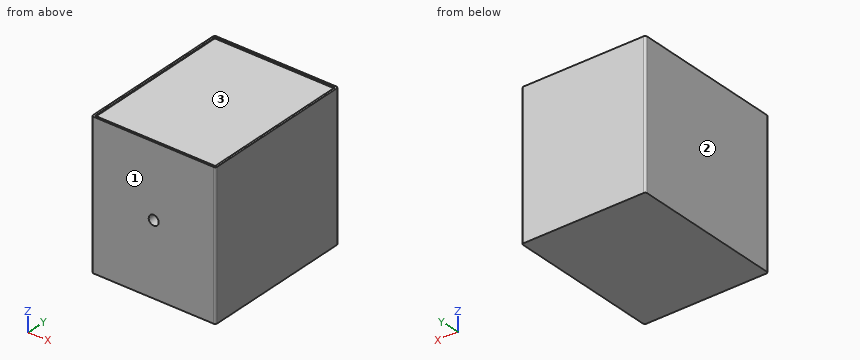
from build123d import *

# Parameters (mm, degrees)
SKETCH1_W                  = 125
SKETCH1_H                  = 155
BOSS_EXTRUDE1_DEPTH        = 145
SKETCH2_W                  = 121
SKETCH2_H                  = 151
CUT_EXTRUDE1_DEPTH         = 1
FILLET1_R                  = 2
FILLET2_R                  = 2
F_10_0MM_DOWEL_HOLE1_D     = 10
F_10_0MM_DOWEL_HOLE1_DEPTH = 20
F_10_0MM_DOWEL_HOLE1_TIP   = 3.004303095


with BuildPart() as part:
    # Sketch1 → Boss-Extrude1 (new body)
    with BuildSketch(Plane.XY):
        with Locations((62.5, 77.5)):
            Rectangle(SKETCH1_W, SKETCH1_H)
    extrude(amount=BOSS_EXTRUDE1_DEPTH)

    # Sketch2 → Cut-Extrude1 (cut)
    with BuildSketch(Plane.XY.offset(145)):
        with Locations((62.5, 77.5)):
            Rectangle(SKETCH2_W, SKETCH2_H)
    extrude(amount=-CUT_EXTRUDE1_DEPTH, mode=Mode.SUBTRACT)

    # Fillet1
    fillet1_edges = [part.edges().sort_by_distance(p)[0] for p in [
        (0, 155, 72.5),
        (125, 155, 72.5),
        (0, 0, 72.5),
    ]]
    fillet(fillet1_edges, radius=FILLET1_R)

    # Fillet2
    fillet2_edges = [part.edges().sort_by_distance(p)[0] for p in [
        (125, 0, 72.5),
    ]]
    fillet(fillet2_edges, radius=FILLET2_R)

    # Ø10.0mm Dowel Hole1
    with Locations(Plane(origin=(62.532008196, 0, 72.5), x_dir=(0, 0, -1), z_dir=(0, -1, 0))):
        with Locations((0, 0)):
            Hole(F_10_0MM_DOWEL_HOLE1_D / 2, depth=F_10_0MM_DOWEL_HOLE1_DEPTH)
            with Locations((0, 0, -(F_10_0MM_DOWEL_HOLE1_DEPTH + F_10_0MM_DOWEL_HOLE1_TIP / 2))):  # 118° drill point
                Cone(0, F_10_0MM_DOWEL_HOLE1_D / 2, F_10_0MM_DOWEL_HOLE1_TIP, mode=Mode.SUBTRACT)


solid = part.part
For this review, take the finished solid that the model builds, in its own axes (mm). Face numbers are marked on the shaded views. Round coordinates to 2 decimals unless told otherwise and drop trailing zeros. Answer as CSV lines item,"result".
(1) Mouldability with a two-part tool opening along X and no side actions: class the marked faces 1, 2 and 3 as +X half, -X half, draft (parallel to the pull), parting line (faces both ways), or undercut.
Checked values:
face 1,"draft"
face 2,"-X half"
face 3,"undercut"
(2) Wall thickness on line 1 (X direction, y = 20, z = 73); line 2 (X direction, y = 6.25, z = 72.5); line 3 (Z direction, x = 30, y = 69.5): over which ranges is each line inside the solid? List them lowest first.
Checked values:
line 1,"x = 0 to 57.56, 67.51 to 125"
line 2,"x = 0 to 57.53, 67.53 to 125"
line 3,"z = 0 to 144"
(3) Insertion check: P1, Ø5, axis at x = 37, y = 26, coming from the +Z side. The pin has a flat end and moves straight along its axis. Give the tip position at first contact, or say it passes through.
Checked values:
P1,"stops at z = 144"
